Can you work these out from the model? Positions are in its coordinate system, mm. Face numbers are marked on the shaded views. A direction names the side the tool comes from. Coordinates: 2 decimals unless noted, no trailing zeros. Order: outer loops, then holes, each group sorted by start corner. A loop starts at its lowest first (then second) coordinate and runs counter-clockwise, first axis right, second up. Notation, with made-up numbers: M 58,85 L 81,85 A31 ccw 81,124 Z; hole C 68.5,75.25 d8. An arc over 180 degrees is marked long. Answer as a JSON object with one key per item and string values.
from build123d import *

# Parameters (mm, degrees)
SKETCH2_W          = 1.4
SKETCH2_H          = 1.3
CUT_EXTRUDE1_DEPTH = 1
CIRPATTERN1_COUNT  = 16


with BuildPart() as part:
    # Sketch1 → Revolve1 (revolve)
    with BuildSketch(Plane(origin=(0, 0, 0), x_dir=(0, 0, -1), z_dir=(1, 0, 0))):
        Polygon((1.76, 2.5), (6, 2.5), (6, 1), (3, 1), (3, -2.5), (0.570548961, -11.482894875), (0.295700194, -11.482894875), (1.76, -2.5), align=None)
    revolve(axis=Axis((0, 0, 0), (0, 1, 0)))

    # Sketch2 → Cut-Extrude1 (cut)
    with BuildSketch(Plane(origin=(0, 2.5, 0), x_dir=(1, 0, 0), z_dir=(0, 1, 0))):
        with Locations((0, 5)):
            Rectangle(SKETCH2_W, SKETCH2_H)
    cut_extrude1 = extrude(amount=-CUT_EXTRUDE1_DEPTH, mode=Mode.SUBTRACT)

    # CirPattern1: Cut-Extrude1 ×16 about axis, 2 skipped
    cirpattern1_axis = Axis((0, 0, 0), (0, -1, 0))
    add([cut_extrude1.rotate(cirpattern1_axis, i * 360 / CIRPATTERN1_COUNT) for i in range(1, CIRPATTERN1_COUNT) if i not in (8, 9)], mode=Mode.SUBTRACT)


solid = part.part
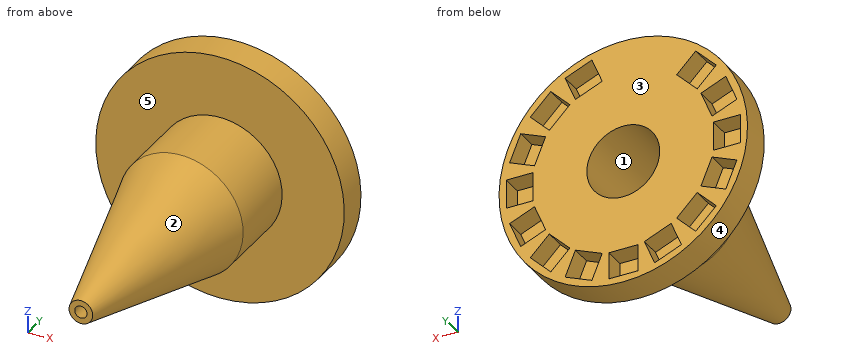
Item 1: If we mould it in two halves opening along X, with no side actions, what happens to the marked faces 1, 2 and 3? For each: pulls with the +X half, pulls with the -X half, needs draft (parallel to the pull), parting line crosses it, or undercut.
Answers follow:
{"face 1": "undercut", "face 2": "parting line crosses it", "face 3": "needs draft"}
Item 2: Which directions (+Z, -Z, +X, -X, +Y, -Y) give clear straight access to the entire face, cutting with the end or side of a thin tool? Please do the marked faces 4 and 5.
Answers follow:
{"face 4": "+Y, -Y", "face 5": "-Y"}
Item 3: I'm going to push flat-ended pins straight in: pin 1 (0.5 mm diameter, centred on x = 4.5, z = 2, fed in from +Y); pin 2 (0.5 mm diameter, centred on x = -5, y = 2, fed in from -Z); pin 3 (3 mm diameter, centred on x = -2.5, y = -4, fed in from +Z). Where does each tip first touch, or does it pass through?
Answers follow:
{"pin 1": "stops at y = 1.5", "pin 2": "stops at z = -3.67", "pin 3": "stops at z = 2.53"}
Item 4: I want a section at C-C, the plane y = 0.25. Write out the boundary of the cut face in (x, z), plus the area to 3 significant figures.
Answers follow:
{"outline": "C 0,0 d6; hole C 0,0 d3.52", "area": "18.5 mm^2"}
Item 5: I want a section at B-B, the plane z = 0. Write out the boundary of the cut face in (x, y).
Answers follow:
{"outline": "M -6,1 L -3,1 L -3,-2.5 L -0.57,-11.48 L -0.3,-11.48 L -1.76,-2.5 L -1.76,2.5 L -4.35,2.5 L -4.35,1.5 L -5.65,1.5 L -5.65,2.5 L -6,2.5 Z; M 0.3,-11.48 L 0.57,-11.48 L 3,-2.5 L 3,1 L 6,1 L 6,2.5 L 5.65,2.5 L 5.65,1.5 L 4.35,1.5 L 4.35,2.5 L 1.76,2.5 L 1.76,-2.5 Z"}
Item 6: I want a section at D-D, the plane x = -4. Write out the boundary of the cut face in (y, z), plus the area to 3 significant figures.
Answers follow:
{"outline": "M 1,-4.47 L 2.5,-4.47 L 2.5,-3.99 L 1.5,-3.99 L 1.5,-3.01 L 2.5,-3.01 L 2.5,-2.41 L 1.5,-2.41 L 1.5,-1.71 L 2.5,-1.71 L 2.5,1.71 L 1.5,1.71 L 1.5,2.41 L 2.5,2.41 L 2.5,3.01 L 1.5,3.01 L 1.5,3.99 L 2.5,3.99 L 2.5,4.47 L 1,4.47 Z", "area": "10.0 mm^2"}
Item 7: I want a section at A-A, the plane x = 0. Write out the boundary of the cut face in (y, z), plus the area to 3 significant figures.
Answers follow:
{"outline": "M -11.48,-0.57 L -2.5,-3 L 1,-3 L 1,-6 L 2.5,-6 L 2.5,-5.65 L 1.5,-5.65 L 1.5,-4.35 L 2.5,-4.35 L 2.5,-1.76 L -2.5,-1.76 L -11.48,-0.3 Z; M -11.48,0.3 L -2.5,1.76 L 2.5,1.76 L 2.5,6 L 1,6 L 1,3 L -2.5,3 L -11.48,0.57 Z", "area": "33.7 mm^2"}
Item 8: Please list where these lines run through material, in increasing order: line 1 (Z direction, x = 0, y = 0.75); line 2 (Y direction, x = 3, z = -2.25).
Answers follow:
{"line 1": "z = -3 to -1.76, 1.76 to 3", "line 2": "y = 1 to 2.5"}
